Read the model definition and answer for the solid it produces. Units are mm, in the model's axes. Face numbers are marked on the shaded views. A direction names the side the tool comes from. Coordinates: 2 decimals unless noted, no trailing zeros. Loops run counter-clockwise (first coordinate to the right, second up) from the corner with the lowest first, then second, coordinate; pieces in that order, holes last. Notation, with made-up numbers: (89, -9) - (110, -9) arc R17 ccw to (110, 20) - close; hole circle Ø7 at (60.5, 52). An arc over 180 degrees is marked (long way). Use CSV: the item, a comma, the result in double quotes.
```python
from build123d import *

# Parameters (mm, degrees)
SZKIC1_R                    = 7.5
SZKIC1_R_2                  = 3.25
DODANIE_WYCI_GNI_CIE1_DEPTH = 4
SZKIC2_R                    = 7.5
SZKIC2_R_2                  = 3.25
DODANIE_WYCI_GNI_CIE2_DEPTH = 2
SZKIC3_R                    = 0.5
DODANIE_WYCI_GNI_CIE3_DEPTH = 2


with BuildPart() as part:
    # Szkic1 → Dodanie-wyciągnięcie1 (new body)
    with BuildSketch(Plane.XY):
        Circle(SZKIC1_R)
        Circle(SZKIC1_R_2, mode=Mode.SUBTRACT)
    extrude(amount=DODANIE_WYCI_GNI_CIE1_DEPTH)

    # Szkic2 → Dodanie-wyciągnięcie2 (add)
    with BuildSketch(Plane.XY.offset(4)):
        Circle(SZKIC2_R)
        Circle(SZKIC2_R_2, mode=Mode.SUBTRACT)
    extrude(amount=DODANIE_WYCI_GNI_CIE2_DEPTH)

    # Szkic3 → Dodanie-wyciągnięcie3 (add)
    with BuildSketch(Plane.XY.offset(6)):
        with Locations((0, 5.5)):
            Circle(SZKIC3_R)
        with Locations((5.5, 0)):
            Circle(SZKIC3_R)
        with Locations((0, -5.5)):
            Circle(SZKIC3_R)
        with Locations((-5.5, 0)):
            Circle(SZKIC3_R)
    extrude(amount=DODANIE_WYCI_GNI_CIE3_DEPTH)


solid = part.part
```
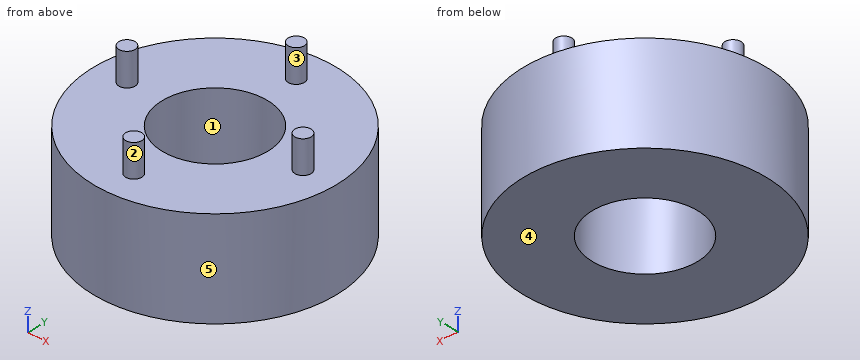
Q1. The part is cut by section C-C on z = 5.5. Determine the outline of the cut face in (x, y).
Reported:
outline,"circle Ø15 at (0, 0); hole circle Ø6.5 at (0, 0)"
Q2. Find the intervals of material crossed by probe 1 along Y at (x, z) = (0, 2.6); probe 2 along Z at (x, y) = (-5.5, -2.5); probe 3 along X at (y, z) = (-1.5, 2.5), in increasing order. Write a range as [from, to].
Reported:
probe 1,"y = [-7.5, -3.25], [3.25, 7.5]"
probe 2,"z = [0, 6]"
probe 3,"x = [-7.35, -2.88], [2.88, 7.35]"
Q3. Given P1, Ø1.5, axis at x = 1.5, z = 7, coming from the -Y side; P2, Ø3, axis at y = -4, z = 5.5, coming from the -X side, each flat-ended and moving along its own axis, determine where each tip first touches the part or whether it passes through.
Reported:
P1,"passes through"
P2,"stops at x = -7.07"
Q4. The part is cut by section D-D on z = 7.25. Determine the outline of the cut face in (x, y), and give its area (3 significant figures).
Reported:
outline,"circle Ø1 at (-5.5, 0); circle Ø1 at (0, -5.5); circle Ø1 at (0, 5.5); circle Ø1 at (5.5, 0)"
area,"3.14 mm²"
Q5. The part is cut by section B-B on y = 2.75. Determine the outline of the cut face in (x, z).
Reported:
outline,"(-6.98, 0) - (-1.73, 0) - (-1.73, 6) - (-6.98, 6) - close; (1.73, 0) - (6.98, 0) - (6.98, 6) - (1.73, 6) - close"
Q6. A tool of negligible diameter and unlimited length cuts with its end or side. For the marked faces 1 and 2, from which of +Z, -Z, +X, -X, +Y, -Y can it reach the whole face along a straight path? Write none if from no direction.
Reported:
face 1,"+Z, -Z"
face 2,"+Z"
Q7. The part is cut by section A-A on x = 0. Determine the outline of the cut face in (y, z), and give its area (3 significant figures).
Reported:
outline,"(-7.5, 0) - (-3.25, 0) - (-3.25, 6) - (-5, 6) - (-5, 8) - (-6, 8) - (-6, 6) - (-7.5, 6) - close; (3.25, 0) - (7.5, 0) - (7.5, 6) - (6, 6) - (6, 8) - (5, 8) - (5, 6) - (3.25, 6) - close"
area,"55.0 mm²"
Q8. For a pull along Y with two mould halves and no side action, classify the marked faces 3, 4 and 5 as +Y half, -Y half, draft (parallel to the pull), parting line (faces both ways), or undercut.
Reported:
face 3,"undercut"
face 4,"draft"
face 5,"parting line"
